Autodesk Inventor part; units mm, degrees
ref_plane "YZ Plane" through (0, 0, 0) normal (1, 0, 0) x (0, 1, 0)
ref_plane "XZ Plane" through (0, 0, 0) normal (0, 1, 0) x (-1, 0, 0)
ref_plane "XY Plane" through (0, 0, 0) normal (0, 0, 1) x (1, 0, 0)
sketch "Sketch1" plane through (0, 0, 0) normal (0, 1, 0) x (-1, 0, 0)
  line L0 (-9.5, 11.5) -> (9.5, 11.5) construction
  line L1 (11.5, 9.5) -> (11.5, -9.5) construction
  line L2 (9.5, -11.5) -> (-9.5, -11.5) construction
  line L3 (-11.5, -9.5) -> (-11.5, 9.5) construction
  line L4 (-11.5, 11.5) -> (11.5, -11.5) construction
  line L5 (11.5, 11.5) -> (-11.5, -11.5) construction
  arc A0 (11.5, 9.5) -> (9.5, 11.5) centre (9.5, 9.5) ccw construction
  arc A1 (9.5, -11.5) -> (11.5, -9.5) centre (9.5, -9.5) ccw construction
  arc A2 (-11.5, -9.5) -> (-9.5, -11.5) centre (-9.5, -9.5) ccw construction
  arc A3 (-9.5, 11.5) -> (-11.5, 9.5) centre (-9.5, 9.5) ccw construction
  line L6 (-9.5, -12.5) -> (9.5, -12.5)
  arc A4 (9.5, -12.5) -> (12.5, -9.5) centre (9.5, -9.5) ccw
  line L7 (12.5, -9.5) -> (12.5, 9.5)
  arc A5 (12.5, 9.5) -> (9.5, 12.5) centre (9.5, 9.5) ccw
  line L8 (9.5, 12.5) -> (-9.5, 12.5)
  arc A6 (-9.5, 12.5) -> (-12.5, 9.5) centre (-9.5, 9.5) ccw
  line L9 (-12.5, 9.5) -> (-12.5, -9.5)
  arc A7 (-12.5, -9.5) -> (-9.5, -12.5) centre (-9.5, -9.5) ccw
  line L10 (10.5, -9.5) -> (10.5, 9.5)
  arc A8 (10.5, 9.5) -> (9.5, 10.5) centre (9.5, 9.5) ccw
  line L11 (9.5, 10.5) -> (-9.5, 10.5)
  arc A9 (-9.5, 10.5) -> (-10.5, 9.5) centre (-9.5, 9.5) ccw
  line L12 (-10.5, 9.5) -> (-10.5, -9.5)
  arc A10 (-10.5, -9.5) -> (-9.5, -10.5) centre (-9.5, -9.5) ccw
  line L13 (-9.5, -10.5) -> (9.5, -10.5)
  arc A11 (9.5, -10.5) -> (10.5, -9.5) centre (9.5, -9.5) ccw
  point P0 (0, 0)
  point P1 (0, 0)
  point P2 (0, 0)
  dimension "d10" = 2
  dimension "depth" = 25
  dimension "width" = 25
  dimension "thickness" = 2
extrude "Extrusion1" add sketch "Sketch1" along normal blind 300
sketch "Sketch2" plane through (12.5, 0, 9.5) normal (1, 0, 0) x (0, 0, -1)
  line L0 (9.5, -60) -> (9.5, 360) construction
  line L1 (0, 300) -> (19, 300)
  line L2 (0, 0) -> (19, 0)
  line L3 (-3, 0) -> (-3, 300)
  line L4 (-3, 150) -> (-40.443, 150) construction
  point P0 (9.5, 0)
  point P1 (9.5, 250)
  point P2 (9.5, 200)
  point P3 (9.5, 50)
  point P4 (9.5, 100)
  dimension "d17" = 50
  dimension "d28" = 50
  dimension "d29" = 100
hole "Hole1" at (12.5, 250, 0) at (12.5, 200, 0) at (12.5, 100, 0) at (12.5, 50, 0) direction (-1, 0, 0) diameter 6.647 depth 20.2 tip angle 118
equation "\"d10\" = thickness"
properties part number "Lacznik prosty" material "Steel"
Check sheet for the modelled part. Datum: model origin and axes. Units: mm. A direction names the side the tool comes from. Round coordinates to 2 decimals unless told otherwise and drop trailing zeros. Order: outer loops, then holes, each group sorted by start corner. A loop starts at its lowest first (then second) coordinate and runs counter-clockwise, first axis right, second up.
(1) Cross-section at D-D, the plane y = 250. Enter the section's corners in (x, z).
(2) Cross-section at C-C, the plane y = 37. Enter the section's corners in (x, z).
(3) Scan lines: probe 1 along Y at (x, z) = (11.7, 0); probe 2 along X at (y, z) = (121, -3). Record each from-to range of solid material in increasing order.
(4) Cross-section at A-A, the plane z = 0. Enter the section's corners in (x, y), and give its area (3 significant figures).
(5) Access from +Z, -Z, +X, -X, +Y, -Y to the whole of each face (thin tool, end or side, straight path). Record for faces 4 (the flat face through (0, 148, 12.5)), 5 (the cylindrical face through (11.486, 253.244, 0.72)), 6 (the flat face through (0, 148, -10.5)).
(6) Draft check along Y on faces 1 (the cylindrical face through (11.486, 53.244, 0.72)), 2 (the flat face through (11, 300, 0)), 3 (the flat face through (-12.5, 148, 0)). Enter one of: pulls with the +Y half, pulls with the -Y half, needs draft (parallel to the pull), parting line crosses it, or undercut.
(7) Cross-section at B-B, the plane x = 4. Enter the section's corners in (y, z).
(8) Go/stop test with a flat-tipped pin: P1, Ø7.5, axis at y = 250, z = 0, coming from the +X side. Record where the tip stops, or that it passes through.
Check sheet entries:
1. outline: (-12.5, -9.5) arc R3 ccw to (-9.5, -12.5) - (9.5, -12.5) arc R3 ccw to (12.5, -9.5) - (12.5, -3.32) - (10.5, -3.32) - (10.5, -9.5) arc R1 cw to (9.5, -10.5) - (-9.5, -10.5) arc R1 cw to (-10.5, -9.5) - (-10.5, 9.5) arc R1 cw to (-9.5, 10.5) - (9.5, 10.5) arc R1 cw to (10.5, 9.5) - (10.5, 3.32) - (12.5, 3.32) - (12.5, 9.5) arc R3 ccw to (9.5, 12.5) - (-9.5, 12.5) arc R3 ccw to (-12.5, 9.5) - close
2. outline: (-12.5, -9.5) arc R3 ccw to (-9.5, -12.5) - (9.5, -12.5) arc R3 ccw to (12.5, -9.5) - (12.5, 9.5) arc R3 ccw to (9.5, 12.5) - (-9.5, 12.5) arc R3 ccw to (-12.5, 9.5) - close; hole (-10.5, -9.5) arc R1 ccw to (-9.5, -10.5) - (9.5, -10.5) arc R1 ccw to (10.5, -9.5) - (10.5, 9.5) arc R1 ccw to (9.5, 10.5) - (-9.5, 10.5) arc R1 ccw to (-10.5, 9.5) - close
3. probe 1: y = 0 to 46.68, 53.32 to 96.68, 103.32 to 196.68, 203.32 to 246.68, 253.32 to 300
3. probe 2: x = -12.5 to -10.5, 10.5 to 12.5
4. outline: (-12.5, 0) - (-10.5, 0) - (-10.5, 300) - (-12.5, 300) - close; (10.5, 0) - (12.5, 0) - (12.5, 46.68) - (10.5, 46.68) - close; (10.5, 53.32) - (12.5, 53.32) - (12.5, 96.68) - (10.5, 96.68) - close; (10.5, 103.32) - (12.5, 103.32) - (12.5, 196.68) - (10.5, 196.68) - close; (10.5, 203.32) - (12.5, 203.32) - (12.5, 246.68) - (10.5, 246.68) - close; (10.5, 253.32) - (12.5, 253.32) - (12.5, 300) - (10.5, 300) - close
4. area: 1,150 mm2
5. face 4: +Z, +X, -X, +Y, -Y
5. face 5: +X
5. face 6: +Y, -Y
6. face 1: undercut
6. face 2: pulls with the +Y half
6. face 3: needs draft
7. outline: (0, -12.5) - (300, -12.5) - (300, -10.5) - (0, -10.5) - close; (0, 10.5) - (300, 10.5) - (300, 12.5) - (0, 12.5) - close
8. P1: stops at x = 12.5
